Geometry check sheet. Reference: the model listing, model coordinates, mm. A direction names the side the tool comes from. Give positions to 0.01 mm unless a question says otherwise; leave off trailing zeros. Write each loop counter-clockwise with the first axis right and the second up, starting at its lowest first coordinate (ties: lowest second). Pieces come first, ordered by that corner, then holes. Notation, with made-up numbers: (-32, 61) - (9, 61) arc R21 cw to (9, 76) - close; hole circle Ø10 at (53, 81.25). An arc over 180 degrees is marked (long way). Write item = value, one per line. Start each with the question number.
(1) Section check C-C, the plane y = 3. Enter the section's corners in (x, z).
(2) Access from +Z, -Z, +X, -X, +Y, -Y to the whole of each face (thin tool, end or side, straight path). Record for faces 5 (the flat face through (-135, -25, 97)), 6 (the flat face through (-164.628, 26, 125)), 7 (the flat face through (-107, 55, 232)), 8 (the flat face through (-109.628, -17, 231)).
(3) Section check B-B, the plane x = -120.5. Enter the section's corners in (y, z).
(4) Section check D-D, the plane z = 201.5. Enter the section's corners in (x, y).
(5) Thickness scan on L1, parallel to X at y = 43.25, z = 17; L2, parallel to Y at x = -148.5, z = 84; L3, parallel to Z at x = -86, y = 55.5. Record the ranges inside material, lowest first.
(6) Draft check along Z on faces 1 (the flat face through (-43, 11, 0)), 2 (the flat face through (-82, 56, 11)), 3 (the flat face through (-98.628, 55, 15)), 4 (the flat face through (-83, 58, 25)). Enter one of: pulls with the +Z half, pulls with the -Z half, needs draft (parallel to the pull), parting line crosses it, or undercut.
(7) Depth check by flat-ended pin: pin 1 Ø10 at (x, y) = (-46.5, 20) entering from +Z; pin 2 Ø4 at (x, z) = (-101.5, 54.5) entering from -Y; pin 3 Ø6.5 at (y, z) = (51, 15.5) entering from -X; pin 4 Ø4 at (x, y) = (-10, -29) entering from -Z. Enter the tip coordinate at first touch or a pass-through.
(8) Section check A-A, the plane z = 229.5. Enter the section's corners in (x, y), plus the area to 3 significant figures.
Autodesk Inventor part; units mm, degrees
ref_plane "Work Plane2" through (-200, 75, 0) normal (0, 1, 0) x (1, 0, 0)
ref_plane "YZ Plane" through (0, 0, 0) normal (1, 0, 0) x (0, 1, 0)
ref_plane "XZ Plane" through (0, 0, 0) normal (0, 1, 0) x (-1, 0, 0)
sketch "Sketch1" plane through (0, 0, 0) normal (0, 0, 1) x (1, 0, 0)
  line L0 (200, 75) -> (-200, 75)
  line L1 (-200, 75) -> (-200, -75)
  line L2 (-200, -75) -> (200, -75)
  line L3 (200, -75) -> (200, 75)
  line L4 (200, 75) -> (-200, -75) construction
  line L5 (-200, 75) -> (200, -75) construction
  point P0 (0, 0)
  dimension "d0" = 400
  dimension "d1" = 150
extrude "Extrusion1" add sketch "Sketch1" along normal blind 2
sketch "Sketch2" plane through (0, 0, 2) normal (0, 0, 1) x (1, 0, 0)
  line L0 (-200, 0) -> (-155, 56.4222) construction
  line L1 (-155, -56.4222) -> (-200, 0) construction
  line L2 (-104.6282, 75) -> (-164.6282, 75)
  line L3 (-164.6282, 75) -> (-164.6282, -25)
  line L4 (-164.6282, -25) -> (-104.6282, -25)
  line L5 (-104.6282, -25) -> (-104.6282, 75)
  line L6 (-104.6282, 75) -> (-164.6282, -25) construction
  line L7 (-164.6282, 75) -> (-104.6282, -25) construction
  line L8 (200, 75) -> (-200, 75)
  point P0 (0, 0)
  point P1 (-134.6282, 25)
  dimension "d5" = 60
  dimension "d6" = 100
  dimension "d55" = 0
extrude "Extrusion2" add sketch "Sketch2" along normal blind 250
sketch "Sketch3" plane through (-104.6282, -25, 2) normal (1, 0, 0) x (0, 0, -1)
  line L0 (0, 0) -> (-250, 0)
  line L1 (0, -50) -> (0, 100)
  line L2 (0, 100) -> (-250, 100)
  line L3 (-250, 0) -> (-250, 100)
  line L4 (0, 20) -> (-150, 20)
  line L5 (-150, 80) -> (0, 80)
  line L6 (0, 20) -> (0, 80)
  line L7 (-150, 80) -> (-150, 20)
  point P0 (2, 25)
  dimension "d27" = 20
  dimension "d28" = 20
extrude "Extrusion3" cut sketch "Sketch3" against normal blind 300 contours L4 L7 L5 L1
sketch "Sketch4" plane through (-104.6282, -25, 252) normal (1, 0, 0) x (0, 0, -1)
  line L0 (0, 100) -> (0, 0)
  line L1 (0, 80) -> (45, 80)
  line L2 (45, 80) -> (45, 15)
  line L3 (0, 15) -> (0, 80)
  line L4 (45, 15) -> (0, 15)
  line L5 (0, 0) -> (0, 100)
  line L6 (0, 15) -> (0, 80)
  point P0 (252, 25)
  dimension "d30" = 65
  dimension "d31" = 15
  dimension "d32" = 45
  dimension "d37" = 65
extrude "Extrusion4" cut sketch "Sketch4" against normal blind 55
sketch "Sketch6" plane through (-104.6282, 55, 207) normal (0, -1, 0) x (1, 0, 0)
  line L0 (0, 0) -> (0, 45)
  line L1 (0, 0) -> (-55, 0)
  line L2 (-55, 0) -> (-55, 45)
  line L3 (0, 45) -> (-55, 45)
  line L4 (-55, 45) -> (0, 45)
  line L5 (0, 45) -> (0, 0)
  line L6 (-5, 45) -> (-5, 0)
  line L7 (-55, 45) -> (-5, 45)
  line L8 (-55, 0) -> (-5, 0)
  line L9 (-55, 45) -> (-55, 0)
  point P0 (104.6282, -207)
  dimension "d40" = 5
extrude "Extrusion5" cut sketch "Sketch6" against normal blind 18 contours L1 L2 L3 L6
sketch "Sketch7" plane through (-104.6282, -10, 252) normal (0, 1, 0) x (1, 0, 0)
  line L0 (-55, 0) -> (-5, 0)
  line L1 (-55, 45) -> (-55, 0)
  line L2 (-5, 45) -> (-55, 45)
  line L3 (-5, 0) -> (-5, 45)
  line L4 (-5, 0) -> (-55, 0)
  line L5 (-55, 0) -> (-55, 45)
  line L6 (-55, 45) -> (-5, 45)
  line L7 (-5, 45) -> (-5, 0)
  point P0 (104.6282, 252)
extrude "Extrusion6" cut sketch "Sketch7" against normal through all
sketch "Sketch10" plane through (-159.6282, -25, 252) normal (1, 0, 0) x (0, 0, -1)
  line L0 (45, 98) -> (0, 98)
  line L1 (45, 98) -> (45, 0)
  line L2 (39.864, 98) -> (45, 0)
  line L3 (45, 0) -> (45, 98)
  line L4 (0, 80) -> (0, 100)
  line L5 (45, 98) -> (39.864, 98)
  point P0 (252, 25)
  dimension "d50" = 3
extrude "Extrusion7" add sketch "Sketch10" along normal blind 55
fillet "Fillet3" radius 2 3 edges at (-109.6282, 73, 232.068) (-109.6282, -17.5, 207.3931) (-109.6282, 64, 211.6643)
sketch "Sketch11" plane through (0, 0, 2) normal (0, 0, 1) x (1, 0, 0)
  line L0 (-104.6282, -5) -> (-104.6282, 55)
  point P0 (0, 0)
  point P1 (-104.6282, 75)
sketch "Sketch12" plane through (-104.6282, -25, 252) normal (1, 0, 0) x (0, 0, -1)
  line L0 (250, 20) -> (100, 20)
  line L1 (100, 80) -> (250, 80)
  arc A0 (100, 80) -> (100, 20) centre (100, 50) ccw
  line L2 (247, 20) -> (250, 20)
  line L3 (247, 80) -> (250, 80)
  line L4 (250, -50) -> (250, 100)
  point P0 (252, 25)
  point P1 (250, 22.1792)
  point P2 (250, 77.8208)
  dimension "d57" = 3
extrude "Extrusion8" add sketch "Sketch12" against normal blind 60
ref_plane "Work Plane2" through (-200, 75, 0) normal (0, 1, 0) x (1, 0, 0)
sketch "Sketch15" plane through (-200, 75, 0) normal (0, 1, 0) x (1, 0, 0)
  line L0 (95.3718, -2) -> (95.3718, -252)
  line L1 (400, -2) -> (95.3718, -2)
  line L2 (100.3718, -11) -> (100.3718, -19)
  line L3 (106.3718, -25) -> (128.3718, -25)
  line L4 (134.3718, -19) -> (134.3718, -11)
  arc A0 (128.3718, -25) -> (134.3718, -19) centre (128.3718, -19) ccw
  arc A1 (100.3718, -19) -> (106.3718, -25) centre (106.3718, -19) ccw
  line L5 (134.3718, -11) -> (100.3718, -11)
  line L6 (100.3718, -11) -> (134.3718, -11)
  line L7 (134.3718, -11) -> (134.3718, -2)
  line L8 (134.3718, -2) -> (100.3718, -2)
  line L9 (100.3718, -2) -> (100.3718, -11)
  point P0 (200, 0)
  point P1 (100.3718, -25)
  point P2 (134.3718, -25)
  dimension "d78" = 14
  dimension "d79" = 34
  dimension "d80" = 6
  dimension "d81" = 5
extrude "Extrusion10" add sketch "Sketch15" against normal blind 35 contours L4 A0 L3 A1 L2 L5
sketch "Sketch16" plane through (-200, 40, 0) normal (0, -1, 0) x (1, 0, 0)
  line L0 (128.3718, 25) -> (106.3718, 25)
  arc A0 (134.3718, 19) -> (128.3718, 25) centre (128.3718, 19) ccw
  arc A1 (106.3718, 25) -> (100.3718, 19) centre (106.3718, 19) ccw
  line L1 (134.3718, 11) -> (134.3718, 19)
  arc A2 (134.3718, 19) -> (128.3718, 25) centre (128.3718, 19) ccw
  line L2 (128.3718, 25) -> (106.3718, 25)
  arc A3 (106.3718, 25) -> (100.3718, 19) centre (106.3718, 19) ccw
  line L3 (100.3718, 19) -> (100.3718, 11)
  line L4 (133.3718, 19) -> (133.3718, 3)
  line L5 (133.3718, 3) -> (101.3718, 3)
  line L6 (101.3718, 3) -> (101.3718, 19)
  arc A4 (106.3718, 24) -> (101.3718, 19) centre (106.3718, 19) ccw
  line L7 (106.3718, 24) -> (128.3718, 24)
  arc A5 (133.3718, 19) -> (128.3718, 24) centre (128.3718, 19) ccw
  line L8 (100.3718, 11) -> (134.3718, 11)
  point P0 (200, 0)
  dimension "d85" = 1
extrude "Extrusion11" cut sketch "Sketch16" against normal blind 31 contours L8 L6 A4 L7 A5 L4 | L4 L5 L6 L8
fillet "Fillet4" radius 3 1 edges at (-200, -75, 1)
fillet "Fillet5" radius 3 1 edges at (-200, 75, 1)
fillet "Fillet6" radius 3 2 edges at (200, -75, 1) (200, 75, 1)
sketch "Sketch18" plane through (200, -72, 0) normal (1, 0, 0) x (0, 0, -1)
  line L0 (-2, 144) -> (0, 144)
  line L1 (-2, 0) -> (-2, 144)
  line L2 (0, 0) -> (-2, 0)
  line L3 (0, 0) -> (0, 144)
  line L4 (-2, 147) -> (-2, 144)
  line L5 (-2, 144) -> (0, 144)
  line L6 (0, 144) -> (0, 147)
  line L7 (0, 147) -> (-2, 147)
  line L8 (-2, 0) -> (-2, -3)
  line L9 (-2, -3) -> (0, -3)
  line L10 (0, -3) -> (0, 0)
  line L11 (0, 0) -> (-2, 0)
  point P0 (0, 72)
extrude "Extrusion12" cut sketch "Sketch18" against normal blind 50
sketch "Sketch19" plane through (-197, -75, 0) normal (0, -1, 0) x (1, 0, 0)
  line L0 (347, 0) -> (347, 2)
  line L1 (0, 2) -> (347, 2)
  line L2 (0, 0) -> (0, 2)
  line L3 (0, 0) -> (347, 0)
  line L4 (0, 2) -> (-3, 2)
  line L5 (-3, 2) -> (-3, 0)
  line L6 (-3, 0) -> (0, 0)
  line L7 (0, 0) -> (0, 2)
  point P0 (197, 0)
extrude "Extrusion13" cut sketch "Sketch19" against normal blind 20
fillet "Fillet7" radius 3 2 edges at (150, -55, 1) (150, 75, 1)
fillet "Fillet8" radius 3 1 edges at (-200, -55, 1)
sketch "Sketch20" plane through (-200, 75, 0) normal (0, 1, 0) x (1, 0, 0)
  line L0 (134.3718, -11) -> (134.3718, -19)
  line L1 (347, -2) -> (95.3718, -2)
  line L2 (134.3718, -11) -> (100, -11)
  line L3 (100, -11) -> (100, -2)
  line L4 (100, -2) -> (134.3718, -2)
  line L5 (134.3718, -2) -> (134.3718, -11)
  point P0 (200, 0)
sketch "Sketch21" plane through (-65.6282, 75, 19) normal (1, 0, 0) x (0, 0, -1)
  line L0 (0, -35) -> (8, -35)
  line L1 (17, -100) -> (17, 0)
  line L2 (8, -35) -> (17, -35)
  line L3 (17, -35) -> (17, 0)
  line L4 (17, 0) -> (8, 0)
  line L5 (8, 0) -> (8, -35)
  point P0 (19, -75)
  point P1 (17, -22.1792)
extrude "Extrusion14" add sketch "Sketch21" against normal blind 37.5
sketch "Sketch22" plane through (-103.1282, 75, 11) normal (0, 0, 1) x (1, 0, 0)
  point P0 (103.1282, -75)
sketch "Sketch23" plane through (-103.1282, 75, 11) normal (0, 0, 1) x (1, 0, 0)
  line L0 (3.5, 0) -> (0, 0)
  line L1 (0, 0) -> (3.5, 0)
  line L2 (3.5, 0) -> (3.5, -35)
  line L3 (3.5, -35) -> (0, -35)
  line L4 (0, -35) -> (0, 0)
  line L5 (37.5, 0) -> (41, 0)
  line L6 (41, 0) -> (41, -35)
  line L7 (41, -35) -> (37.5, -35)
  line L8 (37.5, -35) -> (37.5, 0)
  line L9 (37.5, 0) -> (37.5, -35)
  point P0 (103.1282, -75)
  dimension "d100" = 3.5
  dimension "d101" = 0
sketch "Sketch24" plane through (-200, 40, 0) normal (0, -1, 0) x (1, 0, 0)
  line L0 (133.3718, 11) -> (101.3718, 11)
  line L1 (117.3718, 11) -> (117.3718, 2) construction
  line L2 (134.3718, 2) -> (96.8718, 2)
  line L3 (134.3718, 19) -> (134.3718, 2)
  line L4 (134.3718, 11) -> (134.3718, 2)
  line L5 (100.3718, 11) -> (100.3718, 2)
  line L6 (96.8718, 11) -> (100.3718, 11)
  line L7 (100.3718, 11) -> (100.3718, 2)
  line L8 (100.3718, 2) -> (96.8718, 2)
  line L9 (96.8718, 2) -> (96.8718, 11)
  point P0 (200, 0)
  point P1 (96.8718, 2)
extrude "Extrusion17" cut sketch "Sketch24" against normal through all
sketch "Sketch26" plane through (-200, 40, 0) normal (0, -1, 0) x (1, 0, 0)
  line L0 (101.3718, 11) -> (101.3718, 19)
  line L1 (101.3718, 17) -> (103.3718, 17)
  line L2 (133.3718, 11) -> (101.3718, 11)
  circle A0 centre (103.3718, 17) radius 2
  line L3 (133.3718, 17) -> (131.6357, 17)
  circle A1 centre (103.3718, 17) radius 1.25
  line L4 (103.3718, 18.25) -> (101.3718, 18.25)
  line L5 (101.3718, 18.25) -> (101.3718, 15.75)
  line L6 (101.3718, 15.75) -> (103.3718, 15.75)
  line L7 (103.3718, 15.75) -> (103.3718, 18.25)
  circle A2 centre (130.6718, 17) radius 2
  circle A3 centre (130.6718, 17) radius 1.25
  line L8 (133.3718, 19) -> (133.3718, 11)
  line L9 (130.6718, 18.25) -> (133.3718, 18.25)
  line L10 (133.3718, 18.25) -> (133.3718, 15.25)
  line L11 (133.3718, 15.25) -> (130.6718, 15.25)
  line L12 (130.6718, 15.25) -> (130.6718, 18.25)
  point P0 (200, 0)
  point P1 (132.233, 18.25)
  point P2 (131.64, 15.25)
  point P3 (101.8105, 15.75)
  point P4 (101.8105, 18.25)
  dimension "d116" = 2.5
  dimension "d118" = 2.5
  dimension "d119" = 27.3
  dimension "d112" = 6
  dimension "d113" = 4
  dimension "d117" = 4
extrude "Extrusion18" add sketch "Sketch26" against normal blind 10
extrude "Extrusion19" cut sketch "Sketch26" against normal blind 10 contours A1 L7 L1 | L1 L7 A1 | L7 A1 | A3 L12 | L12 A3
thread "Thread3"
thread "Thread4"
sketch "Sketch28" plane through (150, -72, 0) normal (1, 0, 0) x (0, 0, -1)
  line L0 (0, 144) -> (0, 20)
  line L1 (-2, 20) -> (0, 20)
  line L2 (0, 20) -> (0, 144)
  line L3 (0, 144) -> (-2, 144)
  line L4 (-2, 144) -> (-2, 20)
  point P0 (0, 72)
extrude "Extrusion21" add sketch "Sketch28" along normal blind 50
sketch "Sketch29" plane through (0, 0, 2) normal (0, 0, 1) x (1, 0, 0)
  line L0 (200, 72) -> (200, -52)
  line L1 (200, 72) -> (200, -52)
  line L2 (200, 10) -> (160.5, 10)
  line L3 (160.5, 10) -> (160.5, 16)
  line L4 (160.5, 16) -> (115.5, 16)
  line L5 (115.5, 16) -> (115.5, 4)
  line L6 (115.5, 4) -> (160.5, 4)
  line L7 (160.5, 4) -> (160.5, 16)
  point P0 (0, 0)
  dimension "d136" = 39.5
  dimension "d137" = 6
  dimension "d138" = 45
  dimension "d139" = 12
sketch "Sketch31" plane through (0, 0, 2) normal (0, 0, 1) x (1, 0, 0)
  line L0 (147, 75) -> (-65.6282, 75)
  line L1 (119.1362, 75) -> (234.7266, 75)
  line L2 (234.7266, 75) -> (234.7266, -58.1498)
  line L3 (234.7266, -58.1498) -> (119.1362, -58.1498)
  line L4 (119.1362, -58.1498) -> (119.1362, 75)
  point P0 (0, 0)
extrude "Extrusion24" cut sketch "Sketch31" against normal blind 10
properties part number "lifting base" material "PPS Plastic"
Model answer:
q1.outline = (-200, 0) - (119.14, 0) - (119.14, 2) - (-104.63, 2) - (-104.63, 208.47) - (-159.63, 208.47) - (-159.63, 252) - (-164.63, 252) - (-164.63, 2) - (-200, 2) - close
q2.face_5 = +Z, +X, -X, -Y
q2.face_6 = +Z, -X, +Y, -Y
q2.face_7 = +Z, +X
q2.face_8 = +Z, -Y
q3.outline = (-55, 0) - (75, 0) - (75, 252) - (73, 252) - (73, 212.14) - (-25, 207) - (-25, 2) - (-55, 2) - close
q4.outline = (-164.63, -25) - (-104.63, -25) - (-104.63, 75) - (-164.63, 75) - close
q5.L1 = -164.63 to -104.63, -99.63 to -97.88, -95.38 to -94.63, -71.33 to -70.58, -68.08 to -65.63
q5.L2 = -25 to 75
q5.L3 = 0 to 11, 24 to 25
q6.face_1 = pulls with the -Z half
q6.face_2 = undercut
q6.face_3 = undercut
q6.face_4 = pulls with the +Z half
q7.pin_1 = 2
q7.pin_2 = through
q7.pin_3 = -164.63
q7.pin_4 = 0
q8.outline = (-164.63, -25) - (-159.63, -25) - (-159.63, 73) - (-111.63, 73) arc R2 cw to (-109.63, 71) - (-109.63, 55) - (-104.63, 55) - (-104.63, 75) - (-164.63, 75) - close; (-109.63, -25) - (-104.63, -25) - (-104.63, -10) - (-109.63, -10) - close
q8.area = 776 mm²
